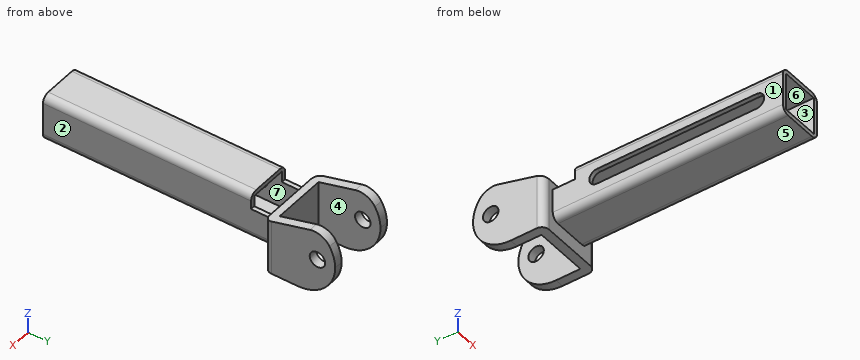
from build123d import *

# Parameters (mm, degrees)
F0_W      = 33.3375
F0_H      = 33.3502
F0_W_2    = 26.9875
F0_H_2    = 27.0002
F1_DEPTH  = 165.1
F2_W      = 15.875
F2_H      = 11.1125
F3_DEPTH  = 33.3385
F5_DEPTH  = 26.9875
F7_DEPTH  = 50.801
F8_R      = 5.08
F9_R      = 12.7
F11_D     = 11.1125
F13_DEPTH = 3.175


with BuildPart() as f1:
    # F0 (on Front) → F1 (new body)
    with BuildSketch(Plane.XZ):
        Rectangle(F0_W, F0_H)
        Rectangle(F0_W_2, F0_H_2, mode=Mode.SUBTRACT)
    extrude(amount=-F1_DEPTH)

    # F2 (on face) → F3 (cut, through all)
    with BuildSketch(Plane(origin=(-16.66875, 0, 0), x_dir=(0, -1, 0), z_dir=(-1, 0, 0))):
        with Locations((-157.1625, 11.11885)):
            Rectangle(F2_W, F2_H)
    extrude(amount=-F3_DEPTH, mode=Mode.SUBTRACT)

    # F4 (on Top) → F5 (join, symmetric)
    with BuildSketch(Plane.XY):
        Polygon((-25.4, 165.1), (25.4, 165.1), (25.4, 215.9), (19.05, 215.9), (19.05, 171.45), (-19.05, 171.45), (-19.05, 215.9), (-25.4, 215.9), align=None)
    extrude(amount=F5_DEPTH, both=True)

    # F6 (on face) → F7 (cut, through all)
    with BuildSketch(Plane(origin=(-25.4, 0, 0), x_dir=(0, -1, 0), z_dir=(-1, 0, 0))):
        with BuildLine():
            ThreePointArc((-215.9, -7.09e-08), (-213.0223149727, 12.1260866825), (-205.002956628, 21.6661570601))
            Line((-205.002956628, 21.6661570601), (-165.1, 11.1125))
            Line((-165.1, 11.1125), (-165.1, 26.9875))
            Line((-165.1, 26.9875), (-215.9, 26.9875))
            Line((-215.9, 26.9875), (-215.9, -7.09e-08))
        make_face()
        with BuildLine():
            ThreePointArc((-188.9125, -26.9875), (-207.9955442322, -19.0830442823), (-215.9, -7.09e-08))
            Line((-215.9, -7.09e-08), (-215.9, -26.9875))
            Line((-215.9, -26.9875), (-188.9125, -26.9875))
        make_face()
    extrude(amount=-F7_DEPTH, mode=Mode.SUBTRACT)

    # F8
    f8_edges = [f1.edges().sort_by_distance(p)[0] for p in [
        (-25.4, 165.1, -7.9375),
        (25.4, 165.1, -7.9375),
        (-16.66875, 74.6125, 16.6751),
        (16.66875, 74.6125, 16.6751),
        (-16.66875, 82.55, -16.6751),
        (16.66875, 82.55, -16.6751),
    ]]
    fillet(f8_edges, radius=F8_R)

    # F9
    f9_edges = [f1.edges().sort_by_distance(p)[0] for p in [
        (22.225, 205.002957, 21.666157),
        (-22.225, 205.002957, 21.666157),
    ]]
    fillet(f9_edges, radius=F9_R)

    # F11 (through all)
    with Locations(Plane(origin=(-25.4, 0, 0), x_dir=(0, -1, 0), z_dir=(-1, 0, 0))):
        with Locations((-203.2, 0)):
            Hole(F11_D / 2)

    # F12 (on face) → F13 (cut, through all)
    with BuildSketch(Plane(origin=(-16.66875, 0, 0), x_dir=(0, -1, 0), z_dir=(-1, 0, 0))):
        with BuildLine():
            Line((-19.05, 5.55625), (-133.35, 5.55625))
            ThreePointArc((-133.35, 5.55625), (-138.90625, 0), (-133.35, -5.55625))
            Line((-133.35, -5.55625), (-19.05, -5.55625))
            ThreePointArc((-19.05, -5.55625), (-13.49375, 0), (-19.05, 5.55625))
        make_face()
    extrude(amount=-F13_DEPTH, mode=Mode.SUBTRACT)


solid = f1.part
Could you check a few things on this model? Use its own coordinates, in mm. Face numbers are marked on the shaded views. A direction names the side the tool comes from. Give positions to 0.01 mm unless a question says otherwise; leave off trailing zeros. Order: outer loops, then holes, each group sorted by start corner. A loop starts at its lowest first (then second) coordinate and runs counter-clockwise, first axis right, second up.
1. Suppose I cut it at C-C (z = 8.5). List the corners of the cut face in (x, y) for me (3 decimals).
2. I need wall thicknesses on L1, parallel to X at y = 26.5, z = -10.5; L2, parallel to X at y = 205.5, z = -15; L3, parallel to Z at x = 1.5, y = 33. Which ranges of each line are inside material? Lowest first, please.
3. Will these pins go through, and if not, where does the flat tip stop? P1, Ø4, axis at x = 10, y = 123.5, coming from the -Z side; P2, Ø1.6, axis at x = -14.5, y = 87.5, coming from the -Z side; P3, Ø4, axis at y = 137.5, z = -16.5, coming from the -X side.
4. Suppose I cut it at B-B (y = 82). List the corners of the cut face in (x, z) for me.
5. We'd pull the mould along Z, two halves only. Please class the marked faces 4, 5, 6 and 7: pulls with the +Z half, pulls with the -Z half, needs draft (parallel to the pull), parting line crosses it, or undercut.
6. For the marked faces 1, 2 and 3, which set-ups out of +Z, -Z, +X, -X, +Y, -Y let a thin tool reach every point of the face, with its end or its side?
7. Suppose I cut it at D-D (y = 203.2). List the corners of the cut face in (x, z) for me.
Solved:
1. outline: (-25.4, 170.18) arc R5.08 ccw to (-20.32, 165.1) - (20.32, 165.1) arc R5.08 ccw to (25.4, 170.18) - (25.4, 214.526) - (19.05, 214.526) - (19.05, 171.45) - (-19.05, 171.45) - (-19.05, 214.526) - (-25.4, 214.526) - close; (-16.669, 0) - (-13.494, 0) - (-13.494, 149.225) - (-16.669, 149.225) - close; (13.494, 0) - (16.669, 0) - (16.669, 149.225) - (13.494, 149.225) - close
2. L1: x = -16.67 to -13.49, 13.49 to 16.67
2. L2: x = -25.4 to -19.05, 19.05 to 25.4
2. L3: z = -16.68 to -13.5, 13.5 to 16.68
3. P1: stops at z = -16.68
3. P2: stops at z = -16.22
3. P3: stops at x = -15.76
4. outline: (-16.67, -11.6) arc R5.08 ccw to (-11.59, -16.68) - (11.59, -16.68) arc R5.08 ccw to (16.67, -11.6) - (16.67, 11.6) arc R5.08 ccw to (11.59, 16.68) - (-11.59, 16.68) arc R5.08 ccw to (-16.67, 11.6) - (-16.67, 5.56) - (-13.49, 5.56) - (-13.49, 13.5) - (13.49, 13.5) - (13.49, -13.5) - (-13.49, -13.5) - (-13.49, -5.56) - (-16.67, -5.56) - close
5. face 4: needs draft
5. face 5: pulls with the -Z half
5. face 6: undercut
5. face 7: undercut
6. face 1: +Z, -Z, -X, -Y
6. face 2: +Z, -Z, +X, -Y
6. face 3: -Y
7. outline: (-25.4, -22.9) - (-19.05, -22.9) - (-19.05, -5.56) - (-25.4, -5.56) - close; (-25.4, 5.56) - (-19.05, 5.56) - (-19.05, 20.01) - (-25.4, 20.01) - close; (19.05, -22.9) - (25.4, -22.9) - (25.4, -5.56) - (19.05, -5.56) - close; (19.05, 5.56) - (25.4, 5.56) - (25.4, 20.01) - (19.05, 20.01) - close
